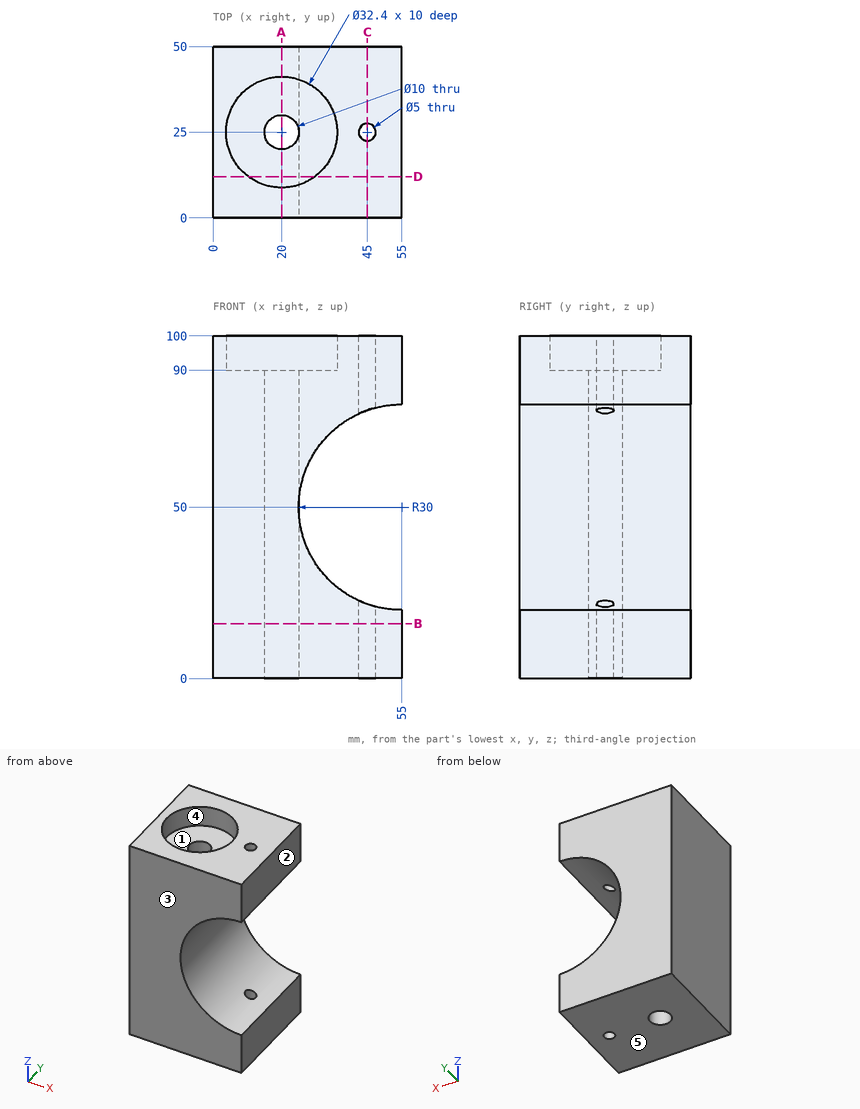
Verification items for this drawing (mm, ordinates from the low corner). A direction names the side the tool comes from. Round coordinates to 2 decimals unless told otherwise and drop trailing zeros. Order: outer loops, then holes, each group sorted by start corner. A loop starts at its lowest first (then second) coordinate and runs counter-clockwise, first axis right, second up. Notation, with made-up numbers: M -3,-17 L 18,-17 A25 ccw 18,9 Z; hole C 5.25,10.25 d1. An arc over 180 degrees is marked long. Answer in a Markdown table with one row per item. Add a question column.
Item 1: Depth check by flat-ended pin: pin 1 Ø4.5 at (x, y) = (45, 25) entering from -Z; pin 2 Ø1 at (x, y) = (16, 29.5) entering from +Z; pin 3 Ø5 at (y, z) = (25, 62) entering from -X. Enter the tip coordinate at first touch or a pass-through.
Item 2: Material ranges on L1, parallel to X at y = 25, z = 15; L2, parallel to X at y = 25, z = 97.25; L3, parallel to Y at x = 20, z = 93.5, recorded low to high. Write a range as [from, to].
Item 3: Draft check along Y on the marked faces 1, 2 and 3. Enter one of: released by +Y, released by -Y, zero draft, split by the parting line, or undercut.
Item 4: Sectioned sample at B-B, the plane z = 16. Enter the section's corners in (x, y).
Item 5: Sectioned sample at A-A, the plane x = 20. Enter the section's corners in (y, z), plus the area to 3 significant figures.
Item 6: Sectioned sample at C-C, the plane x = 45. Enter the section's corners in (y, z), plus the area to 3 significant figures.
Item 7: Set-up check for the marked faces 4 and 5: record each of +Z, -Z, +X, -X, +Y, -Y from which the full face is reachable in a straight line by a thin tool's end or side.
Item 8: Sectioned sample at D-D, the plane y = 12. Enter the section's corners in (x, z), plus the area to 3 significant figures.
Filled in:
| question | item | result |
|---|---|---|
| 1 | pin 1 | passes through |
| 1 | pin 2 | stops at z = 90 |
| 1 | pin 3 | stops at x = 0 |
| 2 | L1 | x = [0, 15], [25, 42.5], [47.5, 55] |
| 2 | L2 | x = [0, 3.8], [36.2, 42.5], [47.5, 55] |
| 2 | L3 | y = [0, 8.8], [41.2, 50] |
| 3 | face 1 | undercut |
| 3 | face 2 | zero draft |
| 3 | face 3 | released by -Y |
| 4 | outline | M 0,0 L 55,0 L 55,50 L 0,50 Z; hole C 20,25 d10; hole C 45,25 d5 |
| 5 | outline | M 0,0 L 20,0 L 20,90 L 8.8,90 L 8.8,100 L 0,100 Z; M 30,0 L 50,0 L 50,100 L 41.2,100 L 41.2,90 L 30,90 Z |
| 5 | area | 3,780 mm² |
| 6 | outline | M 0,0 L 22.5,0 L 22.5,21.72 L 0,21.72 Z; M 0,78.28 L 22.5,78.28 L 22.5,100 L 0,100 Z; M 27.5,0 L 50,0 L 50,21.72 L 27.5,21.72 Z; M 27.5,78.28 L 50,78.28 L 50,100 L 27.5,100 Z |
| 6 | area | 1,950 mm² |
| 7 | face 4 | +Z |
| 7 | face 5 | -Z, +X, -X, +Y, -Y |
| 8 | outline | M 0,0 L 55,0 L 55,20 A30 cw 55,80 L 55,100 L 29.67,100 L 29.67,90 L 10.33,90 L 10.33,100 L 0,100 Z |
| 8 | area | 3,890 mm² |
